Input: part model. Units: mm. Frame: model coordinates. A direction names the side the tool comes from. Give positions to 0.01 mm unless a question says otherwise; leave off trailing zeros. Loops run counter-clockwise (first coordinate to the right, second up) from the corner with the lowest first, then second, coordinate; pieces in that order, holes last. Notation, with made-up numbers: (-31, 19) -> (14, 19) arc R17 ccw to (14, 34) -> close; hole circle Ø7 at (59, 77). An arc over 180 degrees is marked (long way). One line per question, with ' | ' between items.
from build123d import *

# Parameters (mm, degrees)
SKETCH_1_W             = 23.5
SKETCH_1_H             = 12
EXTRUDE_1_DEPTH        = 75
HOLE_WIZARD_M6_1_D     = 5
HOLE_WIZARD_M6_1_DEPTH = 19
HOLE_WIZARD_M6_1_TIP   = 1.502151548
HOLE_WIZARD_M6_2_D     = 5
HOLE_WIZARD_M6_2_DEPTH = 19
HOLE_WIZARD_M6_2_TIP   = 1.502151548


with BuildPart() as part:
    # 草图1 → 凸台-拉伸1 (new, symmetric)
    with BuildSketch(Plane(origin=(0, 0, 0), x_dir=(0, 0, -1), z_dir=(1, 0, 0))):
        Polygon((-15, 15), (-11.5, 15), (-11.5, 13.5), (-11, 13.5), (-11, 12), (-9.5, 12), (-9.5, 15), (-8, 15), (-8, 12.5), (-5, 12.5), (-5, 15), (5, 15), (5, 12.5), (8, 12.5), (8, 15), (9.5, 15), (9.5, 12), (11, 12), (11, 13.5), (11.5, 13.5), (11.5, 15), (15, 15), (15, 8), (12.5, 8), (12.5, 5), (15, 5), (15, -5), (12.5, -5), (12.5, -8), (15, -8), (15, -15), (11.5, -15), (11.5, -13.5), (11, -13.5), (11, -12), (9.5, -12), (9.5, -15), (8, -15), (8, -12.5), (5, -12.5), (5, -15), (-5, -15), (-5, -12.5), (-8, -12.5), (-8, -15), (-9.5, -15), (-9.5, -12), (-11, -12), (-11, -13.5), (-11.5, -13.5), (-11.5, -15), (-15, -15), align=None)
        with BuildLine():
            Line((12, -10.5), (12, -8.5))
            ThreePointArc((12, -8.5), (11.853553391, -8.146446609), (11.5, -8))
            Line((11.5, -8), (-11.5, -8))
            ThreePointArc((-11.5, -8), (-11.853553391, -8.146446609), (-12, -8.5))
            Line((-12, -8.5), (-12, -10.5))
            ThreePointArc((-12, -10.5), (-11.853553391, -10.853553391), (-11.5, -11))
            Line((-11.5, -11), (11.5, -11))
            ThreePointArc((11.5, -11), (11.853553391, -10.853553391), (12, -10.5))
        make_face(mode=Mode.SUBTRACT)
        with BuildLine():
            Line((-11.5, 11), (11.5, 11))
            ThreePointArc((11.5, 11), (11.853553391, 10.853553391), (12, 10.5))
            Line((12, 10.5), (12, 8.5))
            ThreePointArc((12, 8.5), (11.853553391, 8.146446609), (11.5, 8))
            Line((11.5, 8), (-11.5, 8))
            ThreePointArc((-11.5, 8), (-11.853553391, 8.146446609), (-12, 8.5))
            Line((-12, 8.5), (-12, 10.5))
            ThreePointArc((-12, 10.5), (-11.853553391, 10.853553391), (-11.5, 11))
        make_face(mode=Mode.SUBTRACT)
        Rectangle(SKETCH_1_W, SKETCH_1_H, mode=Mode.SUBTRACT)
    extrude(amount=EXTRUDE_1_DEPTH, both=True)

    # M6 螺纹孔1
    with Locations(Plane(origin=(0, 15, 0), x_dir=(1, 0, 0), z_dir=(0, 1, 0))):
        with Locations((-40, 0), (-55, 0), (55, 0), (40, 0)):
            Hole(HOLE_WIZARD_M6_1_D / 2, depth=HOLE_WIZARD_M6_1_DEPTH)
            with Locations((0, 0, -(HOLE_WIZARD_M6_1_DEPTH + HOLE_WIZARD_M6_1_TIP / 2))):  # 118° drill point
                Cone(0, HOLE_WIZARD_M6_1_D / 2, HOLE_WIZARD_M6_1_TIP, mode=Mode.SUBTRACT)

    # M6 螺纹孔2
    with Locations(Plane(origin=(0, -15, 0), x_dir=(-1, 0, 0), z_dir=(0, -1, 0))):
        with Locations((-39, 0), (39, 0)):
            Hole(HOLE_WIZARD_M6_2_D / 2, depth=HOLE_WIZARD_M6_2_DEPTH)
            with Locations((0, 0, -(HOLE_WIZARD_M6_2_DEPTH + HOLE_WIZARD_M6_2_TIP / 2))):  # 118° drill point
                Cone(0, HOLE_WIZARD_M6_2_D / 2, HOLE_WIZARD_M6_2_TIP, mode=Mode.SUBTRACT)


solid = part.part
1. Ray query, line 1 along Y through (x, z) = (-28, 10.5); line 2 along Y through (x, z) = (21.5, 2.5); line 3 along Z through (x, y) = (18, 12.75). Return the intervals inside material, ascending. Write a range as from..to.
Determined:
line 1: y = -12..-11, -8..-6, 6..8, 11..12 | line 2: y = -15..-11, -8..-6, 6..8, 11..15 | line 3: z = -15..-11, -9.5..-8, -5..5, 8..9.5, 11..15
2. Section query C-C (z = 0). Count the separate pieces of the cut face and the enclosed holes in it, then the cut area to 3 significant figures.
Determined:
separate pieces: 16 | enclosed holes: 0 | area: 1,620 mm2
3. Section query A-A (y = -2.25). Output: boundary loops of the cut face in (x, z).
Determined:
outline: (-75, -15) -> (75, -15) -> (75, -11.75) -> (-75, -11.75) -> close; (-75, 11.75) -> (75, 11.75) -> (75, 15) -> (-75, 15) -> close
4. Pin query (flat end, axial travel): P1, Ø8, axis at y = 4, z = 5.5, coming from the +X side; P2, Ø1.5, axis at x = -13.5, z = -6.5, coming from the +Y side. Return the tip coordinate at first contact, or that it passes through.
Determined:
P1: stops at x = 75 | P2: stops at y = 12.5
5. Section query B-B (z = 6.25). Output: boundary loops of the cut face in (x, y), then the cut area to 3 significant figures.
Determined:
outline: (-75, -12.5) -> (75, -12.5) -> (75, -11) -> (-75, -11) -> close; (-75, -8) -> (75, -8) -> (75, -6) -> (-75, -6) -> close; (-75, 6) -> (75, 6) -> (75, 8) -> (-75, 8) -> close; (-75, 11) -> (75, 11) -> (75, 12.5) -> (-75, 12.5) -> close | area: 1,050 mm2
6. Pull-direction query (Z, two-part tool) for faces 5 (the flat face through (1, 12.5, -6)), 6 (the flat face through (1, 8, -14)), 7 (the flat face through (1, 12, -15)); classes: pulls with the +Z half, pulls with the -Z half, needs draft (parallel to the pull), parting line crosses it, or undercut.
Determined:
face 5: undercut | face 6: needs draft | face 7: pulls with the -Z half
7. Reachability of faces 1 (the flat face through (1, 5, -14)), 2 (the cylindrical face through (-42.31, 12.97, 0.96)), 3 (the cylindrical face through (41.31, -12.97, 0.96)), 4 (the flat face through (1, 14, 5)) from +Z, -Z, +X, -X, +Y, -Y: full face, straight path, thin tool, end or side. Return the list, or none.
Determined:
face 1: -Z, +X, -X | face 2: +Y | face 3: -Y | face 4: +X, -X, +Y
